Can you work these out from the model? Positions are in its coordinate system, mm. A direction names the side the tool comes from. Give positions to 0.01 mm unless a question says otherwise; leave off trailing zeros. Order: outer loops, then holes, each group sorted by start corner. A loop starts at its lowest first (then second) coordinate and runs counter-clockwise, first axis right, second up. Notation, with made-up numbers: (11.5, -34) - (67.5, -34) arc R21 ccw to (67.5, -8) - close; hole circle Ø1 at (-7, 82). An arc over 180 degrees is marked (long way). Use one line per item in the form item = value. Start each with the question number.
1) Suppose I cut it at A-A, the plane x = 12.7. Write out the boundary of the cut face in (y, z) (1 decimal).
2) Which directions (+Z, -Z, +X, -X, +Y, -Y) give clear straight access to the entire face, cutting with the end or side of a thin tool? Please do faces 5 (the flat face through (92, 10.16, 20)), 6 (the flat face through (47, 16, 25.4)), 7 (the cylindrical face through (88.811, 24.193, 17.233)), 8 (the flat face through (51, 27.94, 2)), 9 (the flat face through (95.25, 4, 16)).
3) Please list where these lines run through material, in increasing order: probe 1 along X at (y, z) = (9, 19.05); probe 2 along X at (y, z) = (10, 20.5); probe 3 along X at (y, z) = (11.5, 9.75).
4) Suppose I cut it at D-D, the plane x = 69. Write out the boundary of the cut face in (y, z) (3 decimals).
5) Suppose I cut it at B-B, the plane z = 8. Write out the boundary of the cut face in (x, y) (3 decimals), and give its area (3 significant figures).
6) For pin 1 (12 mm diameter, centred on x = 18, y = 14, fed in from -Z); pin 2 (3 mm diameter, centred on y = 20, z = 6.5, fed in from +X); pin 3 (4 mm diameter, centred on x = 73, y = 8.5, fed in from -Z), each with a flat end and sliding along its axis, tell me the tip position at first contact or that it passes through.
7) We'd pull the mould along Y, two halves only. Please class faces 1 (the flat face through (88.9, 15, 20)), 2 (the flat face through (47, 0, 13)), 3 (the flat face through (47, 31.115, 13)), 4 (the cylindrical face through (77.75, 15.34, 18.71)): released by +Y, released by -Y, zero draft, split by the parting line, or undercut.
8) Suppose I cut it at C-C, the plane y = 15.5. State how many separate pieces and enclosed holes the cut face has, and give its area (3 significant figures).
Autodesk Inventor part; units mm, degrees
ref_plane "YZ Plane" through (0, 0, 0) normal (1, 0, 0) x (0, 1, 0)
ref_plane "XZ Plane" through (0, 0, 0) normal (0, 1, 0) x (-1, 0, 0)
ref_plane "XY Plane" through (0, 0, 0) normal (0, 0, 1) x (1, 0, 0)
sketch "Sketch1" plane through (0, 0, 0) normal (1, 0, 0) x (0, 1, 0)
  line L0 (0, 0) -> (31.115, 0)
  line L1 (31.115, 0) -> (31.115, 25.4)
  line L2 (31.115, 25.4) -> (0, 25.4)
  line L3 (0, 25.4) -> (0, 0)
  dimension "d0" = 25.4
  dimension "d1" = 31.115
extrude "Extrusion1" add sketch "Sketch1" along normal blind 95.25
sketch "Sketch2" plane through (95.25, 0, 0) normal (1, 0, 0) x (0, 0, -1)
  arc A0 (-3.175, 27.94) -> (-3.175, 2.54) centre (-3.175, 15.24) ccw
  line L0 (0, 0) -> (0, 31.115)
  line L1 (-25.4, 0) -> (0, 0)
  line L2 (-3.175, 27.94) -> (0, 27.94)
  line L3 (-3.175, 2.54) -> (0, 2.54)
  dimension "d4" = 3.175
  dimension "d5" = 15.24
  dimension "d6" = 25.4
extrude "Extrusion2" cut sketch "Sketch2" against normal blind 88.9
sketch "Sketch3" plane through (0, 31.115, 25.4) normal (0, 1, 0) x (1, 0, 0)
  line L0 (0, 25.4) -> (0, 0)
  line L1 (95.25, 25.4) -> (95.25, 0)
  line L2 (0, 0) -> (95.25, 0)
  point P0 (12.7, 6.35)
  point P1 (76.2, 6.35)
  dimension "d9" = 0
  dimension "d10" = 12.7
  dimension "d12" = 6.35
  dimension "d35" = 76.2
hole "Hole1" at (12.7, 31.115, 19.05) at (76.2, 31.115, 19.05) direction (0, -1, 0) diameter 3.175 end through all
sketch "Sketch4" plane through (95.25, 0, 0) normal (1, 0, 0) x (0, 0, -1)
  line L0 (-10.782, 20.32) -> (-30.1642, 20.32)
  line L1 (-30.1642, 20.32) -> (-30.1642, 10.16)
  line L2 (-30.1642, 10.16) -> (-10.782, 10.16)
  line L3 (-10.782, 10.16) -> (-10.782, 20.32)
  line L4 (-25.4, 0) -> (0, 0)
  dimension "d20" = 10.16
  dimension "d21" = 10.16
extrude "Extrusion3" cut sketch "Sketch4" against normal blind 6.35
sketch "Sketch5" plane through (95.25, 0, 0) normal (1, 0, 0) x (0, 0, -1)
  line L0 (-25.4, 10.16) -> (-25.4, 0)
  line L1 (-25.4, 0) -> (0, 0)
  line L2 (-25.4, 31.115) -> (-25.4, 20.32)
  line L3 (0, 31.115) -> (-25.4, 31.115)
  point P0 (-19.05, 24.765)
  point P1 (-19.05, 6.35)
  dimension "d24" = 6.35
  dimension "d25" = 6.35
  dimension "d26" = 6.35
  dimension "d27" = 6.35
hole "Hole2" at (95.25, 24.765, 19.05) at (95.25, 6.35, 19.05) direction (-1, 0, 0) diameter 3.81 depth 12.7 tip angle 118.188
properties part number "bATTERYrAILS"
Result sheet:
q1.outline = (0, 0) - (2.5, 0) - (2.5, 3.2) arc R12.7 cw to (27.9, 3.2) - (27.9, 0) - (31.1, 0) - (31.1, 17.5) - (0, 17.5) - close; (0, 20.6) - (31.1, 20.6) - (31.1, 25.4) - (0, 25.4) - close
q2.face_5 = +Z, -Z, +X
q2.face_6 = +Z, +X, -X, +Y, -Y
q2.face_7 = +X
q2.face_8 = -Z, +X
q2.face_9 = +Z, -Z, +X, +Y, -Y
q3.probe_1 = 0 to 11.11, 14.29 to 74.61, 77.79 to 95.25
q3.probe_2 = 0 to 12.05, 13.35 to 75.55, 76.85 to 95.25
q3.probe_3 = 0 to 6.35
q4.outline = (0, 0) - (2.54, 0) - (2.54, 3.175) arc R12.7 cw to (27.94, 3.175) - (27.94, 0) - (31.115, 0) - (31.115, 25.4) - (0, 25.4) - close
q5.outline = (0, 0) - (95.25, 0) - (95.25, 3.492) - (6.35, 3.492) - (6.35, 26.988) - (95.25, 26.988) - (95.25, 31.115) - (0, 31.115) - close
q5.area = 875 mm²
q6.pin_1 = 13.61
q6.pin_2 = 6.35
q6.pin_3 = 12.39
q7.face_1 = undercut
q7.face_2 = released by -Y
q7.face_3 = released by +Y
q7.face_4 = zero draft
q8.separate_pieces = 1
q8.enclosed_holes = 2
q8.area = 932 mm²
